from build123d import *

# Parameters (mm, degrees)
PLATE_BODY_DEPTH          = 2
SKETCH2_R                 = 4.0238
SHAFT_BEARINGS_DEPTH      = 95.22122903
SLOT_DEPTH                = 95.22122903
SKETCH5_R                 = 1.25
BOLT_HOLES_DEPTH          = 95.22122903
SKETCH6_W                 = 0.5
SKETCH6_H                 = 40
CUT_EXTRUDE1_DEPTH        = 95.22122903
SKETCH8_W                 = 3
SKETCH8_H                 = 5
FINGER_JOINTS_DEPTH       = 2
SKETCH9_W                 = 10
SKETCH9_H                 = 20
GEAR_HOLE_DEPTH           = 97.756601842
CUT_EXTRUDE3_DEPTH        = 10
F_1MM_FILLETS_GEAR_HOLE_R = 1
F_7MM_FILLET_GEAR_HOLE_R  = 7


with BuildPart() as part:
    # Sketch1 → plate_body (new body)
    with BuildSketch(Plane.XY):
        Polygon((0, 40), (0, 0), (33.935876329, 0), (47, -11), (50, -11), (50, -51), (79.2, -51), (79.2, 10), (52, 10), (52, 40), align=None)
    extrude(amount=PLATE_BODY_DEPTH)

    # Sketch2 → shaft_bearings (cut, through all)
    with BuildSketch(Plane.XY.offset(2)):
        with Locations((6, 20)):
            Circle(SKETCH2_R)
        with Locations((44, 20)):
            Circle(SKETCH2_R)
    extrude(amount=-SHAFT_BEARINGS_DEPTH, mode=Mode.SUBTRACT)

    # Sketch4 → slot (cut, through all)
    with BuildSketch(Plane.XY.offset(2)):
        with BuildLine():
            Line((26.425, 34), (26.425, 6))
            ThreePointArc((26.425, 6), (25, 4.575), (23.575, 6))
            Line((23.575, 6), (23.575, 34))
            ThreePointArc((23.575, 34), (25, 35.425), (26.425, 34))
        make_face()
    extrude(amount=-SLOT_DEPTH, mode=Mode.SUBTRACT)

    # Sketch5 → bolt_holes (cut, through all)
    with BuildSketch(Plane.XY.offset(2)):
        with Locations((3, 37)):
            Circle(SKETCH5_R)
        with Locations((47, 37)):
            Circle(SKETCH5_R)
        with Locations((3, 3)):
            Circle(SKETCH5_R)
    extrude(amount=-BOLT_HOLES_DEPTH, mode=Mode.SUBTRACT)

    # Sketch6 → Cut-Extrude1 (cut, through all)
    with BuildSketch(Plane.XY.offset(2)):
        with Locations((50.25, -31)):
            Rectangle(SKETCH6_W, SKETCH6_H)
    extrude(amount=-CUT_EXTRUDE1_DEPTH, mode=Mode.SUBTRACT)

    # Sketch8 → finger_joints (add)
    with BuildSketch(Plane.XY.offset(2)):
        with Locations((49, -33.5)):
            Rectangle(SKETCH8_W, SKETCH8_H)
        with Locations((49, -43.5)):
            Rectangle(SKETCH8_W, SKETCH8_H)
        with Locations((80.7, -43.5)):
            Rectangle(SKETCH8_W, SKETCH8_H)
        with Locations((80.7, -33.5)):
            Rectangle(SKETCH8_W, SKETCH8_H)
        with Locations((49, -13.5)):
            Rectangle(SKETCH8_W, SKETCH8_H)
        with Locations((49, -23.5)):
            Rectangle(SKETCH8_W, SKETCH8_H)
        with Locations((80.7, -23.5)):
            Rectangle(SKETCH8_W, SKETCH8_H)
        with Locations((80.7, -13.5)):
            Rectangle(SKETCH8_W, SKETCH8_H)
    extrude(amount=-FINGER_JOINTS_DEPTH)

    # Sketch9 → gear_hole (cut, through all)
    with BuildSketch(Plane.XY.offset(2)):
        with Locations((62, -31)):
            Rectangle(SKETCH9_W, SKETCH9_H)
    extrude(amount=-GEAR_HOLE_DEPTH, mode=Mode.SUBTRACT)

    # Sketch12 → Cut-Extrude3 (cut)
    with BuildSketch(Plane.XY.offset(2)):
        Polygon((79.2, 10), (79.2, -3.5), (65.7, 10), align=None)
    extrude(amount=-CUT_EXTRUDE3_DEPTH, mode=Mode.SUBTRACT)

    # 1mm_fillets_gear_hole
    # the kernel refuses this fillet: 1 mm, written as the material it adds along each edge
    with BuildSketch(Plane(origin=(33.935876329, 0, 0), x_dir=(-1, 0, 0), z_dir=(0, 0, 1))) as f_1mm_fillets_gear_hole_piece_1:
        with BuildLine():
            CenterArc((F_1MM_FILLETS_GEAR_HOLE_R * 0.364933095837, F_1MM_FILLETS_GEAR_HOLE_R), F_1MM_FILLETS_GEAR_HOLE_R, 229.902601193, 40.097398807)
            Line((-F_1MM_FILLETS_GEAR_HOLE_R * 0.279155806295, F_1MM_FILLETS_GEAR_HOLE_R * 0.23504935705), (0, 0))
            Line((0, 0), (F_1MM_FILLETS_GEAR_HOLE_R * 0.364933095837, 0))
        make_face()
    extrude(amount=2)
    with BuildSketch(Plane(origin=(47.5, -11, 2), x_dir=(0, -1, 0), z_dir=(0, 0, -1))) as f_1mm_fillets_gear_hole_piece_2:
        with BuildLine():
            CenterArc((0.866025404, 1), F_1MM_FILLETS_GEAR_HOLE_R, 210, 60)
            Line((0, 0.5), (0, 0))
            Line((0, 0), (0.866025404, 0))
        make_face()
    extrude(amount=2)
    # the kernel refuses this fillet: 1 mm, written as the material it takes off along each edge
    with BuildSketch(Plane(origin=(0, 0, -2.5), x_dir=(0, 1, 0), z_dir=(0, 0, 1)), Plane(origin=(50.5, -51, 4.5), x_dir=(1, 0, 0), z_dir=(0, 0, -1))) as f_1mm_fillets_gear_hole_2_piece_1:
        with BuildLine():
            CenterArc((F_1MM_FILLETS_GEAR_HOLE_R, -F_1MM_FILLETS_GEAR_HOLE_R), F_1MM_FILLETS_GEAR_HOLE_R, 90, 90)
            Line((0, -F_1MM_FILLETS_GEAR_HOLE_R), (0, 0))
            Line((0, 0), (F_1MM_FILLETS_GEAR_HOLE_R, 0))
        make_face()
    extrude(amount=7, mode=Mode.SUBTRACT)
    with BuildSketch(Plane(origin=(0, 40, -2.5), x_dir=(0, -1, 0), z_dir=(0, 0, 1)), Plane(origin=(52, 40, -2.5), x_dir=(-1, 0, 0), z_dir=(0, 0, 1)), Plane(origin=(79.2, -51, -2.5), x_dir=(0, 1, 0), z_dir=(0, 0, 1))) as f_1mm_fillets_gear_hole_2_piece_2:
        with BuildLine():
            CenterArc((F_1MM_FILLETS_GEAR_HOLE_R, F_1MM_FILLETS_GEAR_HOLE_R), F_1MM_FILLETS_GEAR_HOLE_R, 180, 90)
            Line((0, F_1MM_FILLETS_GEAR_HOLE_R), (0, 0))
            Line((0, 0), (F_1MM_FILLETS_GEAR_HOLE_R, 0))
        make_face()
    extrude(amount=7, mode=Mode.SUBTRACT)
    with BuildSketch(Plane(origin=(79.2, -3.5, 3.035533906), x_dir=(-0.7071067811865523, 0.7071067811865427, 0), z_dir=(0, 0, -1)), Plane(origin=(65.7, 10, 3.035533906), x_dir=(-1, 0, 0), z_dir=(0, 0, -1))) as f_1mm_fillets_gear_hole_2_piece_3:
        with BuildLine():
            CenterArc((F_1MM_FILLETS_GEAR_HOLE_R * 0.414213562373, -F_1MM_FILLETS_GEAR_HOLE_R), F_1MM_FILLETS_GEAR_HOLE_R, 90, 45)
            Line((-F_1MM_FILLETS_GEAR_HOLE_R * 0.292893218813, -F_1MM_FILLETS_GEAR_HOLE_R * 0.292893218813), (0, 0))
            Line((0, 0), (F_1MM_FILLETS_GEAR_HOLE_R * 0.414213562373, 0))
        make_face()
    extrude(amount=4.071067812, mode=Mode.SUBTRACT)

    # 7mm_fillet_gear_hole
    f_7mm_fillet_gear_hole_edges = [part.edges().sort_by_distance(p)[0] for p in [
        (52, 10, 1),
    ]]
    fillet(f_7mm_fillet_gear_hole_edges, radius=F_7MM_FILLET_GEAR_HOLE_R)


solid = part.part
Read the model definition and answer for the solid it produces. Units are mm, in the model's axes. A direction names the side the tool comes from. Round coordinates to 2 decimals unless told otherwise and drop trailing zeros. Write each loop counter-clockwise with the first axis right and the second up, starting at its lowest first coordinate (ties: lowest second). Pieces come first, ordered by that corner, then holes. Notation, with made-up numbers: M 4,26.25 L 63,26.25 A9 ccw 63,31.25 Z; hole C 10,55 d11. An arc over 180 degrees is marked long. Use a Markdown table: item, result.
1) Straight lines are drawn through the part: line 1 along X through (y, z) = (-29, 1.1); line 2 along Y through (x, z) = (3, 0.5); line 3 along X through (y, z) = (-23, 1.35). For each, find the intervals that lie inside material, in ascending order. Write a range as [from, to].
Answers follow:
| item | result |
|---|---|
| line 1 | x = [50.5, 57], [67, 79.2] |
| line 2 | y = [0, 1.75], [4.25, 17.32], [22.68, 35.75], [38.25, 40] |
| line 3 | x = [47.5, 57], [67, 82.2] |
2) The part is cut by section A-A (y = -39). Write down the section's boundary in (x, z), plus the area to 3 significant figures.
Answers follow:
| item | result |
|---|---|
| outline | M 50.5,0 L 57,0 L 57,2 L 50.5,2 Z; M 67,0 L 79.2,0 L 79.2,2 L 67,2 Z |
| area | 37.4 mm2 |
3) For a pull along X with two mould halves and no side action, classify faces 5 (the flat face through (49, -46, 1)), 6 (the cylindrical face through (4.19, 3.38, 1.01)), 7 (the flat face through (50.5, -39, 1)) as pulls with the +X half, pulls with the -X half, needs draft (parallel to the pull), parting line crosses it, or undercut.
Answers follow:
| item | result |
|---|---|
| face 5 | needs draft |
| face 6 | undercut |
| face 7 | pulls with the -X half |
4) The part is cut by section D-D (z = 1.5). Give the number of separate pieces and of enclosed holes in the cut face, plus the area to 3 significant figures.
Answers follow:
| item | result |
|---|---|
| separate pieces | 1 |
| enclosed holes | 7 |
| area | 3,560 mm2 |
5) The part is cut by section B-B (x = 6). Write down the section's boundary in (y, z), plus the area to 3 significant figures.
Answers follow:
| item | result |
|---|---|
| outline | M 0,0 L 15.98,0 L 15.98,2 L 0,2 Z; M 24.02,0 L 40,0 L 40,2 L 24.02,2 Z |
| area | 63.9 mm2 |
6) The part is cut by section C-C (y = 37). Write down the section's boundary in (x, z).
Answers follow:
| item | result |
|---|---|
| outline | M 0,0 L 1.75,0 L 1.75,2 L 0,2 Z; M 4.25,0 L 45.75,0 L 45.75,2 L 4.25,2 Z; M 48.25,0 L 52,0 L 52,2 L 48.25,2 Z |
7) Flat-ended cylindrical pins translate along their axes: pin 1 (1 mm diameter, centred on x = 13.5, z = 1, fed in from -Y); pin 2 (1 mm diameter, centred on y = 5.5, z = 1.5, fed in from -X); pin 3 (2 mm diameter, centred on x = 47, y = 37, fed in from -Z); pin 4 (1 mm diameter, centred on x = 80, z = 1, fed in from -Y). Find the tip coordinate at first contact, or state that the pin passes through.
Answers follow:
| item | result |
|---|---|
| pin 1 | stops at y = 0 |
| pin 2 | stops at x = 0 |
| pin 3 | passes through |
| pin 4 | stops at y = -46 |
8) A tool of negligible diameter and unlimited length cuts with its end or side. For faces 1 (the flat face through (81, -11, 1)), 2 (the flat face through (67, -31, 1)), 3 (the flat face through (49, -21, 1)), 4 (the flat face through (81, -21, 1)), from which of +Z, -Z, +X, -X, +Y, -Y can it reach the whole face along a straight path? Write none if from no direction.
Answers follow:
| item | result |
|---|---|
| face 1 | +Z, -Z, +X, +Y |
| face 2 | +Z, -Z |
| face 3 | +Z, -Z, -X |
| face 4 | +Z, -Z, +X |
